Autodesk Inventor part; units mm, degrees
ref_plane "YZ Plane" through (0, 0, 0) normal (1, 0, 0) x (0, 1, 0)
ref_plane "XZ Plane" through (0, 0, 0) normal (0, 1, 0) x (-1, 0, 0)
ref_plane "XY Plane" through (0, 0, 0) normal (0, 0, 1) x (1, 0, 0)
sketch "스케치1" plane through (0, 0, 0) normal (0, 0, 1) x (1, 0, 0)
  circle A0 centre (0, 0) radius 20 construction
  circle A1 centre (0, 20) radius 2.3
  circle A2 centre (-19.0211, 6.1803) radius 2.3
  circle A3 centre (-11.7557, -16.1803) radius 2.3
  circle A4 centre (11.7557, -16.1803) radius 2.3
  circle A5 centre (19.0211, 6.1803) radius 2.3
  circle A6 centre (0, 0) radius 25
  dimension "d0" = 40
  dimension "d1" = 4.6
  dimension "d4" = 360
  dimension "d6" = 50
extrude "돌출1" add sketch "스케치1" along normal blind 5
sketch "스케치2" plane through (0, 0, 0) normal (0, 0, -1) x (-1, 0, 0)
  circle A0 centre (0, 0) radius 7.35
  dimension "d9" = 14.7
extrude "돌출2" add sketch "스케치2" along normal blind 10
chamfer "모따기1" distance 0.5 angle 45 5 edges at (-21.3211, 6.1803, 5) (-2.3, 20, 5) (16.7211, 6.1803, 5) (9.4557, -16.1803, 5) (-14.0557, -16.1803, 5)
sketch "스케치3" plane through (0, 0, -10) normal (0, 0, -1) x (-1, 0, 0)
  circle A0 centre (0, 0) radius 7.35
  line L0 (4, 6.1662) -> (4, -6.1662)
  dimension "d15" = 4
extrude "돌출3" cut sketch "스케치3" against normal blind 10 contours A0 L0 picked at (5.1167, 0)
properties part number "회전축 상단"
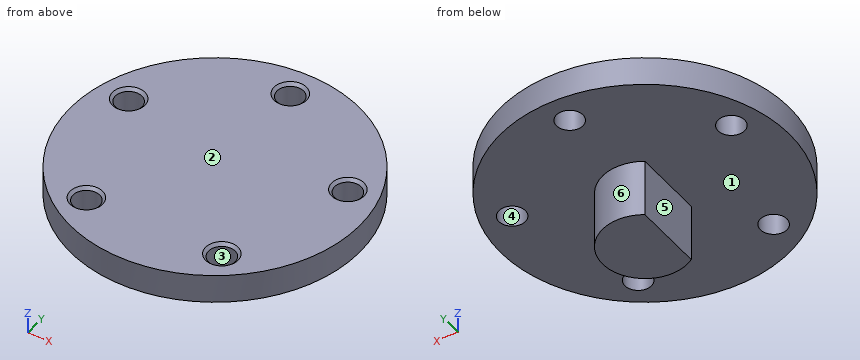
Can you work these out from the model? Positions are in its coordinate system, mm. Face numbers are marked on the shaded views. A direction names the side the tool comes from. Round coordinates to 2 decimals unless told otherwise and drop trailing zeros. Loops run counter-clockwise (first coordinate to the right, second up) from the corner with the lowest first, then second, coordinate; pieces in that order, holes last. Notation, with made-up numbers: M 51,52.25 L 110,52.25 A31 cw 110,86.25 Z; hole C 67.5,68.25 d1. An arc over 180 degrees is marked long. Answer in a Markdown table with one row per item.
1. On a 3-axis mill with a long thin cutter (end or side, diameter ignored), from which of +Z, -Z, +X, -X, +Y, -Y can I reach the whole of each face in a straight line? I mean the marked faces 4, 5 and 6. Say none if no direction works.
Established:
| item | result |
|---|---|
| face 4 | +Z, -Z |
| face 5 | -Z, -X, +Y, -Y |
| face 6 | -Z |
2. If we section it at D-D, the plane x = -7: Please give me the cut outline in (y, z).
Established:
| item | result |
|---|---|
| outline | M -24,0 L 24,0 L 24,5 L -24,5 Z |
3. I'm going to push flat-ended pins straight in: pin 1 Ø2 at (x, y) = (-10.5, 1.5) entering from -Z; pin 2 Ø8 at (x, z) = (-3.5, -3.5) entering from +Y; pin 3 Ø8 at (y, z) = (2.5, -1) entering from +X; pin 4 Ø5 at (y, z) = (-1, -4.5) entering from -X. Where does each tip first touch, or does it pass through?
Established:
| item | result |
|---|---|
| pin 1 | z = 0 |
| pin 2 | y = 24.95 |
| pin 3 | x = 25 |
| pin 4 | x = -4 |
4. Please list where these lines run through material, in increasing order: line 1 (Z direction, x = -6.5, y = -16.5); line 2 (Y direction, x = 0, z = 2.4); line 3 (X direction, y = 18.5, z = 3.5). Write a range as from..to.
Established:
| item | result |
|---|---|
| line 1 | 0..5 |
| line 2 | -25..17.7, 22.3..25 |
| line 3 | -16.82..-1.74, 1.74..16.82 |
5. If we section it at A-A, the plane y = 20: Please give me the cut outline in (x, z).
Established:
| item | result |
|---|---|
| outline | M -15,0 L -2.3,0 L -2.3,4.5 L -2.8,5 L -15,5 Z; M 2.3,0 L 15,0 L 15,5 L 2.8,5 L 2.3,4.5 Z |
6. Thinking about a two-plate mould opening in Z: for the marked faces 1, 2 and 3, which applies, pulls with the +Z half, pulls with the -Z half, needs draft (parallel to the pull), parting line crosses it, or undercut?
Established:
| item | result |
|---|---|
| face 1 | pulls with the -Z half |
| face 2 | pulls with the +Z half |
| face 3 | needs draft |
7. If we section it at B-B, the plane x = 0: Please give me the cut outline in (y, z).
Established:
| item | result |
|---|---|
| outline | M -25,0 L -7.35,0 L -7.35,-10 L 7.35,-10 L 7.35,0 L 17.7,0 L 17.7,4.5 L 17.2,5 L -25,5 Z; M 22.3,0 L 25,0 L 25,5 L 22.8,5 L 22.3,4.5 Z |
8. If we section it at C-C, the plane y = 0: Please give me the cut outline in (x, z), plus the area to 4 significant figures.
Established:
| item | result |
|---|---|
| outline | M -25,0 L -4,0 L -4,-10 L 7.35,-10 L 7.35,0 L 25,0 L 25,5 L -25,5 Z |
| area | 363.5 mm² |
